Could you check a few things on this drawing? It's one solid part, dimensions in mm from its lowest x, y, z. Give positions to 0.01 mm unless a question says otherwise; leave off trailing zeros. Order: outer loops, then holes, each group sorted by start corner. A loop starts at its lowest first (then second) coordinate and runs counter-clockwise, first axis right, second up. Notation, with made-up numbers: (82, 34.5) - (117, 34.5) arc R8 cw to (117, 46.5) - close; hole circle Ø9 at (-31, 18.5). An arc over 180 degrees is marked (long way). Return JSON: item names as keys, results as strings.
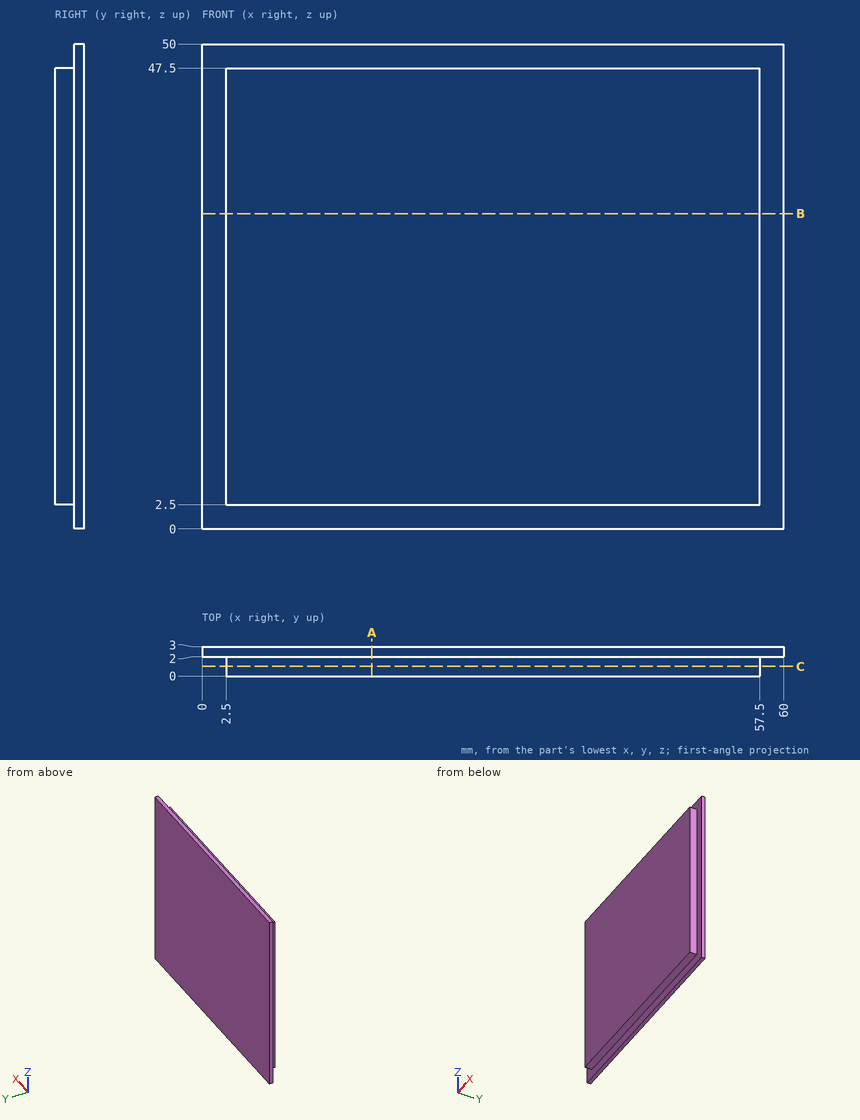
1. Suppose I cut it at B-B (z = 32.5). List the corners of the cut face in (x, y) for me, plus the area to 3 significant figures.
Checks:
{"outline": "(0, 2) - (2.5, 2) - (2.5, 0) - (57.5, 0) - (57.5, 2) - (60, 2) - (60, 3) - (0, 3) - close", "area": "170 mm^2"}
2. For pin 1 Ø1.6 at (y, z) = (1, 29) entering from -X; pin 2 Ø0.6 at (x, y) = (43, 1) entering from -Z; pin 3 Ø1 at (y, z) = (0.5, 36) entering from +X, each with a flat end and sliding along its axis, tell me the tip position at first contact or that it passes through.
Checks:
{"pin 1": "x = 2.5", "pin 2": "z = 2.5", "pin 3": "x = 57.5"}
3. Suppose I cut it at A-A (x = 17.5). List the corners of the cut face in (y, z) for me.
Checks:
{"outline": "(0, 2.5) - (2, 2.5) - (2, 0) - (3, 0) - (3, 50) - (2, 50) - (2, 47.5) - (0, 47.5) - close"}
4. Suppose I cut it at C-C (y = 1). List the corners of the cut face in (x, z) for me.
Checks:
{"outline": "(2.5, 2.5) - (57.5, 2.5) - (57.5, 47.5) - (2.5, 47.5) - close"}
5. If I drill on L1, parallel to Z at x = 23, y = 0.75; L2, parallel to X at y = 1.55, z = 27, over which ranges is the centre line in solid material (lowest first)? Write a range as [from, to].
Checks:
{"L1": "[2.5, 47.5]", "L2": "[2.5, 57.5]"}
